```python
from build123d import *

# Parameters (mm, degrees)
SKETCH022_W             = 1.57
SKETCH022_H             = 3
PAD011_DEPTH            = 0.1
SKETCH024_W             = 0.05
SKETCH024_H             = 1
SKETCH025_W             = 0.05
SKETCH025_H             = 1
SKETCH026_W             = 1.6
SKETCH026_H             = 1.5
PAD012_DEPTH            = 0.05
FILLET004_R             = 0.09
FILLET005_R             = 0.1
FILLET006_R             = 0.04
REVOLUTION001_ANGLE     = 180
SKETCH028_R             = 3
PAD013_DEPTH            = 0.2
SKETCH020_R             = 4
PAD010_DEPTH            = 2.5
SKETCH023_W             = 2.920448
SKETCH023_H             = 7.916798
SKETCH023_W_2           = 3.050448
POCKET004_DEPTH         = 2.501
BODY010_PLACEMENT_ANGLE = 90


with BuildPart() as pad001:
    # Sketch022 → Pad011 (new body)
    with BuildSketch(Plane.XY):
        with Locations((4.415, 0.035576)):
            Rectangle(SKETCH022_W, SKETCH022_H)
    extrude(amount=-PAD011_DEPTH)

    # Sketch024 (on Face6 of Pad011) → AdditiveLoft002 section 0
    with BuildSketch(Plane(origin=(0, 0, -0.1), x_dir=(1, 0, 0), z_dir=(0, 0, -1))):
        with Locations((5.175, -1.035576)):
            Rectangle(SKETCH024_W, SKETCH024_H)
    # Sketch025 (on Face6 of Pad011) → AdditiveLoft002 section 1
    with BuildSketch(Plane(origin=(0, 0, -1.4), x_dir=(1, 0, 0), z_dir=(0, 0, -1))):
        with Locations((5.575, -1.028005)):
            Rectangle(SKETCH025_W, SKETCH025_H)
    loft()

    # Sketch026 (on Face11 of AdditiveLoft002) → Pad012 (join)
    with BuildSketch(Plane(origin=(0, 0, -1.4), x_dir=(1, 0, 0), z_dir=(0, 0, -1))):
        with Locations((6.35, -1.028005)):
            Rectangle(SKETCH026_W, SKETCH026_H)
    extrude(amount=PAD012_DEPTH)

    # Fillet004
    fillet004_edges = [pad001.edges().sort_by_distance(p)[0] for p in [
        (5.2, 0.035576, 0),
    ]]
    fillet(fillet004_edges, radius=FILLET004_R)

    # Fillet005
    fillet005_edges = [pad001.edges().sort_by_distance(p)[0] for p in [
        (5.6, 1.028005, -1.4),
    ]]
    fillet(fillet005_edges, radius=FILLET005_R)

    # Fillet006
    fillet006_edges = [pad001.edges().sort_by_distance(p)[0] for p in [
        (5.55, 1.028005, -1.45),
    ]]
    fillet(fillet006_edges, radius=FILLET006_R)


with BuildPart() as pad001_1:
    # Body008 placement: moved
    add(pad001.part.moved(Location((0, 0, 1))))


with BuildPart() as len001:
    # Sketch021 (on DatumPlane) → Revolution001 (revolve)
    with BuildSketch(Plane.XY.offset(2.5)):
        with BuildLine():
            Line((-3, 0), (3, 0))
            ThreePointArc((3, 0), (0, 3), (-3, 0))
        make_face()
    revolve(axis=Axis((0, 0, 2.5), (1, 0, 0)), revolution_arc=REVOLUTION001_ANGLE)


with BuildPart() as thermalpad001:
    # Sketch028 → Pad013 (new body)
    with BuildSketch(Plane.XY):
        Circle(SKETCH028_R)
    extrude(amount=PAD013_DEPTH)


with BuildPart() as thermalpad001_1:
    # Body009 placement: moved
    add(thermalpad001.part.moved(Location((0, 0, -0.2))))


with BuildPart() as led2:
    # Sketch020 → Pad010 (new body)
    with BuildSketch(Plane.XY):
        Circle(SKETCH020_R)
    extrude(amount=PAD010_DEPTH)

    # Sketch023 (on Face3 of Pad010) → Pocket004 (cut, through all)
    with BuildSketch(Plane.XY.offset(2.5)):
        with Locations((5.090224, -0.060281)):
            Rectangle(SKETCH023_W, SKETCH023_H)
        with Locations((-5.025224, 0.060281)):
            Rectangle(SKETCH023_W_2, SKETCH023_H)
    extrude(amount=-POCKET004_DEPTH, mode=Mode.SUBTRACT)

    # Fusion001: union PAD001, Len001, ThermalPad001
    add(pad001_1.part)
    add(len001.part)
    add(thermalpad001_1.part)


with BuildPart() as led2_1:
    # Fusion001 placement: moved
    add(led2.part.moved(Location((9.2, 28.5, -1))))


with BuildPart() as led2_2:
    # Body010 placement: moved
    add(led2_1.part.moved(Location((58.4, -9.2, 0))).rotate(Axis((58.4, -9.2, 0), (0, 0, 1)), BODY010_PLACEMENT_ANGLE))


solid = led2_2.part
```
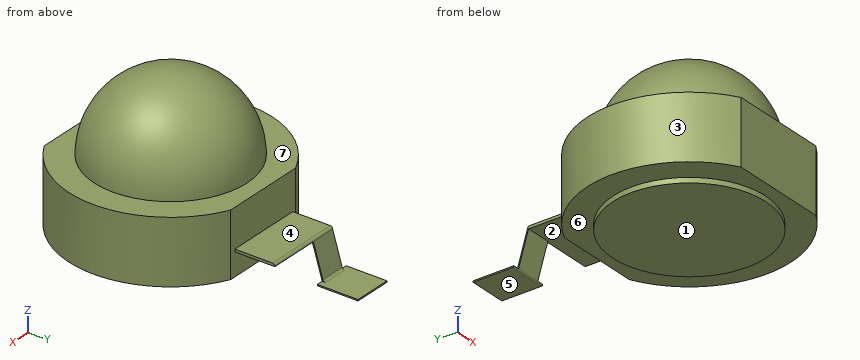
Model file for the job. Use its own axes, mm. Face numbers are marked on the shaded views. A direction names the side the tool comes from. Coordinates: 2 decimals unless noted, no trailing zeros. Write each loop counter-clockwise with the first axis right and the second up, starting at its lowest first coordinate (ties: lowest second). Pieces come first, ordered by that corner, then holes. Notation, with made-up numbers: (24, 52) - (75, 52) arc R15 ccw to (75, 57) - close; hole circle Ø6 at (8.5, 41.5). An arc over 180 degrees is marked (long way). One line per item, written item: value. Start each with the question number.
1. Slice it at D-D (y = -2). Write the cut outline in (x, z), plus the area to 3 significant figures.
2. Slice it at C-C (z = 0.25). Write the cut outline in (x, y), plus the area to 3 significant figures.
3. Slice it at A-A (y = 0). Write the cut outline in (x, z), plus the area to 3 significant figures.
4. Probe line 1 (Z direction, x = 27.5, y = 2); line 2 (Y direction, x = 30, z = -0.3); line 3 (X direction, y = -2, z = 1.55). List the from-to ranges inside material, lowest first. Write a range as from..to.
5. Tool access for the marked faces 4, 5, 6 and 7: list every direction of +Z, -Z, +X, -X, +Y, -Y with a clear straight run to the whole face (end or side of a thin tool).
6. Flat gauge pins, fed straight in: pin 1 (1.5 mm diameter, centred on x = 31, z = 0.5, fed in from +Y); pin 2 (1 mm diameter, centred on x = 32.5, y = 0.5, fed in from -Z); pin 3 (0.8 mm diameter, centred on x = 30, z = 0.5, fed in from +Y). Where does each tip first touch, or does it go through?
7. Mould opens along Y. For the marked faces 1, 2 and 3 say: released by +Y, released by -Y, zero draft, split by the parting line, or undercut.
Answers below:
1. outline: (26.44, -1) - (27.66, -1) - (27.66, -1.2) - (32.14, -1.2) - (32.14, -1) - (33.36, -1) - (33.36, 1.5) - (32.14, 1.5) arc R2.24 ccw to (27.66, 1.5) - (26.44, 1.5) - close
1. area: 26.1 mm^2
2. outline: (27.96, -3.5) - (31.84, -3.5) arc R4 ccw to (31.58, 3.63) - (28.22, 3.63) arc R4 ccw to start
2. area: 48.1 mm^2
3. outline: (25.9, -1) - (26.9, -1) - (26.9, -1.2) - (32.9, -1.2) - (32.9, -1) - (33.9, -1) - (33.9, 1.5) - (32.9, 1.5) arc R3 ccw to (26.9, 1.5) - (25.9, 1.5) - close
3. area: 35.3 mm^2
4. line 1: z = -1..1.5
4. line 2: y = -3.5..3.63
4. line 3: x = 27.66..32.14
5. face 4: +Z, +X, -X, +Y
5. face 5: -Z, +X, -X, +Y, -Y
5. face 6: -Z
5. face 7: +Z
6. pin 1: stops at y = 5.2
6. pin 2: stops at z = -1.2
6. pin 3: stops at y = 3.63
7. face 1: zero draft
7. face 2: undercut
7. face 3: split by the parting line
